Build history of the part. All positions in model axes, mm. A direction names the side the tool comes from. Give positions to 0.01 mm unless a question says otherwise; leave off trailing zeros. Write each loop counter-clockwise with the first axis right and the second up, starting at its lowest first coordinate (ties: lowest second). Pieces come first, ordered by that corner, then holes.
Autodesk Inventor part; units mm, degrees
ref_plane "YZ Plane" through (0, 0, 0) normal (1, 0, 0) x (0, 1, 0)
ref_plane "XZ Plane" through (0, 0, 0) normal (0, 1, 0) x (-1, 0, 0)
ref_plane "XY Plane" through (0, 0, 0) normal (0, 0, 1) x (1, 0, 0)
sketch "Sketch1" plane through (0, 0, 0) normal (0, 0, 1) x (1, 0, 0)
  circle A0 centre (0, 0) radius 6.6 construction
  circle A1 centre (-6.9148, 6.9148) radius 1.5875 construction
  circle A2 centre (6.9148, 6.9148) radius 1.5875 construction
  circle A3 centre (-6.9148, -6.9148) radius 1.5875 construction
  circle A4 centre (6.9148, -6.9148) radius 1.5875 construction
  line L0 (-6.9148, 6.9148) -> (6.9148, 6.9148) construction
  line L1 (6.9148, 6.9148) -> (6.9148, -6.9148) construction
  line L2 (6.9148, -6.9148) -> (-6.9148, -6.9148) construction
  line L3 (-6.9148, -6.9148) -> (-6.9148, 6.9148) construction
  circle A5 centre (0, 0) radius 12.958 construction
  line L4 (-6.9148, -6.9148) -> (6.9148, 6.9148) construction
  line L5 (-6.9148, 6.9148) -> (-5.7923, 5.7923) construction
  line L6 (-5.7923, 5.7923) -> (-4.6669, 4.6669) construction
  line L7 (-8.0373, 8.0373) -> (-9.1627, 9.1627) construction
  circle A6 centre (0, 0) radius 4
  line L8 (0, 4) -> (0, 5.05) construction
  line L9 (0, -20.9412) -> (0, 20.9412) construction
  line L10 (-1.475, 5.05) -> (1.475, 5.05)
  line L11 (-1.475, 5.05) -> (-1.475, 3.7181)
  line L12 (1.475, 5.05) -> (1.475, 3.7181)
  circle A7 centre (0, 0) radius 14.958
  circle A8 centre (6.9148, 6.9148) radius 1.2891
  circle A9 centre (6.9148, -6.9148) radius 1.2891
  circle A10 centre (-6.9148, -6.9148) radius 1.2891
  circle A11 centre (-6.9148, 6.9148) radius 1.2891
  dimension "d0" = 13.2
  dimension "d1" = 3.175
  dimension "d5" = 13.8296
  dimension "d6" = 45
  dimension "d9" = 8
  dimension "d10" = 1.05
  dimension "d11" = 2.95
  dimension "d14" = 2
  dimension "d15" = 29.916
  dimension "d21" = 2.5781
extrude "HubFeature" add sketch "Sketch1" against normal blind 6.5
sketch "Sketch2" plane through (0, 0, 0) normal (0, 0, 1) x (1, 0, 0)
  circle A0 centre (0, 0) radius 6.6
  line L0 (-1.475, 5.05) -> (1.475, 5.05)
  line L1 (-1.475, 3.7181) -> (-1.475, 5.05)
  line L2 (1.475, 5.05) -> (1.475, 3.7181)
  arc A1 (-1.475, 3.7181) -> (1.475, 3.7181) centre (0, 0) ccw
extrude "LipFeature" add sketch "Sketch2" along normal blind 10
sketch "Sketch3" plane through (0, 0, -6.5) normal (0, 0, -1) x (-1, 0, 0)
  circle A0 centre (0, 0) radius 12
  dimension "d18" = 24
extrude "BearingIndentFeature" cut sketch "Sketch3" against normal blind 3.5
sketch "SetScrewHole" plane through (0, 0, 0) normal (1, 0, 0) x (0, 1, 0)
  line L0 (6.6, 10) -> (-6.6, 10) construction
  line L1 (-6.6, 0) -> (6.6, 0) construction
  line L2 (-4, 10) -> (3.7181, 10) construction
  circle A0 centre (0, 6.5) radius 1.25
  line L3 (0, 10) -> (0, 0) construction
  line L4 (14.958, 0) -> (-14.958, 0)
  dimension "d22" = 2.5
  dimension "d25" = 3.5
extrude "SetScrewHoleFeature" cut sketch "SetScrewHole" against normal through all
properties part number "BaseHub"
(1) Drop flat-ended pins along their axis: pin 1 (5 mm diameter, centred on x = -10.5, z = 4, fed in from -Y); pin 2 (1.1 mm diameter, centred on y = 4, z = 2.5, fed in from -X); pin 3 (2 mm diameter, centred on x = 3, z = -4, fed in from +Y); pin 4 (1.5 mm diameter, centred on y = 0, z = 6.5, fed in from -X). Give the stop position or say it passes through.
(2) Saw through at B-B, the plane z = 3.5. List the corners of the cut face in (x, y) (3 decimals), plus the area to 3 significant figures.
(3) Saw through at C-C, the plane z = -0.75. List the corners of the cut face in (x, y) (3 decimals).
(4) 3-axis set-ups, long thin cutter, end or side, ignore diameter. For faces 4 (the face through (6.295, -1.982, 4.93)), 5 (the face through (-1.475, 4, 4)), 6 (the face through (11.99, 0.53, -4.77)): which of +Z, -Z, +X, -X, +Y, -Y reach the whole face in a straight line?
(5) Mould opens along X. For faces 1 (the face through (0, -4, 5)), 2 (the face through (-3.243, -14.602, -3.204)), 3 (the face through (-5.18, -1.25, 6.55)) say: +X half, -X half, draft (parallel to the pull), parting line (faces both ways), or undercut.
(6) Probe line 1 (Y direction, x = 0, z = -4.9); line 2 (Y direction, x = -7.5, z = -1.5); line 3 (X direction, y = -0.25, z = 8). List the from-to ranges inside material, lowest first.
Computed values:
1. pin 1: passes through
1. pin 2: stops at x = -5.63
1. pin 3: stops at y = 14.82
1. pin 4: stops at x = 3.93
2. outline: circle Ø13.2 at (0, 0); hole (-1.475, 3.718) arc R4 ccw (long way) to (1.475, 3.718) - (1.475, 5.05) - (-1.475, 5.05) - close
2. area: 83.2 mm2
3. outline: circle Ø29.916 at (0, 0); hole circle Ø2.578 at (-6.915, -6.915); hole circle Ø2.578 at (-6.915, 6.915); hole (-1.475, 3.718) arc R4 ccw (long way) to (1.475, 3.718) - (1.475, 5.05) - (-1.475, 5.05) - close; hole circle Ø2.578 at (6.915, -6.915); hole circle Ø2.578 at (6.915, 6.915)
4. face 4: +Z
4. face 5: +Z, -Z
4. face 6: -Z
5. face 1: undercut
5. face 2: parting line
5. face 3: draft
6. line 1: y = -14.96 to -12, 12 to 14.96
6. line 2: y = -12.94 to -8.06, -5.77 to 5.77, 8.06 to 12.94
6. line 3: x = -6.6 to -3.99, 3.99 to 6.6
